Read the model definition and answer for the solid it produces. Units are mm, in the model's axes. Face numbers are marked on the shaded views. A direction names the side the tool comes from. Coordinates: 2 decimals unless noted, no trailing zeros. Write each loop counter-clockwise with the first axis right and the second up, starting at its lowest first coordinate (ties: lowest second). Pieces come first, ordered by that corner, then holes. Notation, with made-up numbers: (22, -28.75) -> (60, -28.75) arc R13 ccw to (60, -14.75) -> close; hole circle Ø8 at (88, 6). An arc over 180 degrees is marked (long way). One line per item, written item: value. Start each with the question number.
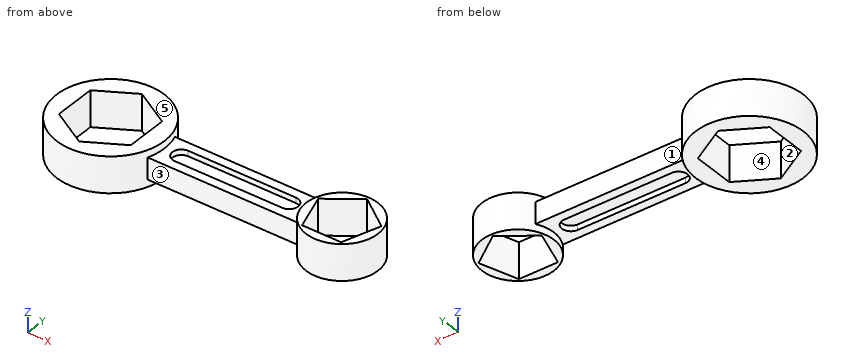
Autodesk Fusion 360 part; units mm, degrees
sketch "Sketch1" plane through (0, 0, 0) normal (0, 0, 1) x (1, 0, 0)
  circle A0 centre (0, 0) radius 30
  circle A1 centre (129, 0) radius 20
  line L0 (0, 23.094) -> (-20, 11.547)
  line L1 (-20, 11.547) -> (-20, -11.547)
  line L2 (-20, -11.547) -> (0, -23.094)
  line L3 (0, -23.094) -> (20, -11.547)
  line L4 (20, -11.547) -> (20, 11.547)
  line L5 (20, 11.547) -> (0, 23.094)
  line L6 (146.6336, 5.7295) -> (129, 18.541)
  line L7 (129, 18.541) -> (111.3664, 5.7295)
  line L8 (111.3664, 5.7295) -> (118.1019, -15)
  line L9 (118.1019, -15) -> (139.8981, -15)
  line L10 (139.8981, -15) -> (146.6336, 5.7295)
  line L11 (28.2843, 10) -> (111.6795, 10)
  line L12 (28.2843, -10) -> (111.6795, -10)
  line L13 (99.5, 5) -> (39.5, 5)
  line L14 (39.5, -5) -> (99.5, -5)
  arc A2 (39.5, 5) -> (39.5, -5) centre (39.5, 0) ccw
  arc A3 (99.5, -5) -> (99.5, 5) centre (99.5, 0) ccw
  point P0 (129, 0)
  point P1 (69.5, 0)
  dimension "d2" = 129
  dimension "d4" = 20
  dimension "d5" = 60
  dimension "d6" = 15
  dimension "d7" = 40
  dimension "d8" = 60
  dimension "d9" = 10
  dimension "d11" = 10
  dimension "d12" = 20
extrude "Extrude1" add sketch "Sketch1" along normal mid plane 20 contours A0 | A1 makes body 1 at (148.9006, -1.9914, -3.3333) makes body 2 at (27.1662, -12.7278, 3.3333)
extrude "Extrude2" add sketch "Sketch1" along normal mid plane 12 contours A0 A1 L11 L12 bodies 1 2
extrude "Extrude3" add sketch "Sketch1" along normal mid plane 6 contours L13 L14 A2 A3 bodies 1
1. For a pull along X with two mould halves and no side action, classify the marked faces 4 and 5 as +X half, -X half, draft (parallel to the pull), parting line (faces both ways), or undercut.
2. A cutting plane is placed at C-C on y = 0. Give the vertices of the cut face in (x, z).
3. A cutting plane is placed at B-B on x = 15. Give the vertices of the cut face in (y, z).
4. A cutting plane is placed at D-D on x = 48.5. Give the vertices of the cut face in (y, z).
5. A cutting plane is placed at A-A on y = 15.5. Give the vertices of the cut face in (x, z).
6. Find the intervals of material crossed by probe 1 along X at (y, z) = (-2, 8.25); probe 2 along X at (y, z) = (16, -4.5); probe 3 along X at (y, z) = (9, 4.5), in increasing order. Write a range as from..to.
7. A tool of negligible diameter and unlimited length cuts with its end or side. For the marked faces 1, 2 and 3, from which of +Z, -Z, +X, -X, +Y, -Y can it reach the whole face along a straight path? Write none if from no direction.
8. Given pin 1 (12 mm diameter, centred on x = 53, z = 1, fed in from -Y); pin 2 (1.5 mm diameter, centred on y = -18, z = -4.5, fed in from -X); pin 3 (2 mm diameter, centred on x = 3.5, z = -2, fed in from -Y); pin 4 (10 mm diameter, centred on x = 66.5, y = -19.5, fed in from -Z), each flat-ended and moving along its own axis, determine where each tip first touches the part or whether it passes through.
Derived:
1. face 4: undercut
1. face 5: draft
2. outline: (-30, -10) -> (-20, -10) -> (-20, 10) -> (-30, 10) -> close; (20, -10) -> (30, -10) -> (30, -6) -> (34.5, -6) -> (34.5, -3) -> (104.5, -3) -> (104.5, -6) -> (109, -6) -> (109, -10) -> (113.23, -10) -> (113.23, 10) -> (109, 10) -> (109, 6) -> (104.5, 6) -> (104.5, 3) -> (34.5, 3) -> (34.5, 6) -> (30, 6) -> (30, 10) -> (20, 10) -> close; (144.77, -10) -> (149, -10) -> (149, 10) -> (144.77, 10) -> close
3. outline: (-25.98, -10) -> (-14.43, -10) -> (-14.43, 10) -> (-25.98, 10) -> close; (14.43, -10) -> (25.98, -10) -> (25.98, 10) -> (14.43, 10) -> close
4. outline: (-10, -6) -> (-5, -6) -> (-5, -3) -> (5, -3) -> (5, -6) -> (10, -6) -> (10, 6) -> (5, 6) -> (5, 3) -> (-5, 3) -> (-5, 6) -> (-10, 6) -> close
5. outline: (-25.69, -10) -> (-13.15, -10) -> (-13.15, 10) -> (-25.69, 10) -> close; (13.15, -10) -> (25.69, -10) -> (25.69, 10) -> (13.15, 10) -> close; (116.36, -10) -> (124.81, -10) -> (124.81, 10) -> (116.36, 10) -> close; (133.19, -10) -> (141.64, -10) -> (141.64, 10) -> (133.19, 10) -> close
6. probe 1: x = -29.93..-20, 20..29.93, 109.1..113.88, 144.12..148.9
6. probe 2: x = -25.38..-12.29, 12.29..25.38, 117..125.5, 132.5..141
6. probe 3: x = -28.62..-20, 20..115.87, 142.13..146.86
7. face 1: +Z, -Z, +Y
7. face 2: +Z, -Z
7. face 3: +Z, -Z, -Y
8. pin 1: stops at y = -10
8. pin 2: stops at x = -24.54
8. pin 3: stops at y = -29.9
8. pin 4: passes through
